Autodesk Inventor part; units mm, degrees
ref_plane "YZ Plane" through (0, 0, 0) normal (1, 0, 0) x (0, 1, 0)
ref_plane "XZ Plane" through (0, 0, 0) normal (0, 1, 0) x (-1, 0, 0)
sketch "Sketch1" plane through (0, 0, 0) normal (0, 0, 1) x (1, 0, 0)
  line L0 (0, 0) -> (98, 0)
  line L1 (98, 0) -> (98, 11.5)
  line L2 (98, 11.5) -> (0, 11.5)
  line L3 (0, 11.5) -> (0, 0)
  circle A0 centre (8, 5.75) radius 4
  arc A1 (7, 4.632) -> (7, 6.868) centre (8, 5.75) ccw
  line L4 (7, 6.868) -> (7, 4.632)
  circle A2 centre (28, 5.75) radius 4
  arc A3 (27, 4.632) -> (27, 6.868) centre (28, 5.75) ccw
  line L5 (27, 6.868) -> (27, 4.632)
  circle A4 centre (48, 5.75) radius 4
  arc A5 (47, 4.632) -> (47, 6.868) centre (48, 5.75) ccw
  line L6 (47, 6.868) -> (47, 4.632)
  circle A6 centre (68, 5.75) radius 4
  arc A7 (67, 4.632) -> (67, 6.868) centre (68, 5.75) ccw
  line L7 (67, 6.868) -> (67, 4.632)
  circle A8 centre (88, 5.75) radius 4
  arc A9 (87, 4.632) -> (87, 6.868) centre (88, 5.75) ccw
  line L8 (87, 6.868) -> (87, 4.632)
  point P0 (0, 5.75)
  dimension "d0" = 11.5
  dimension "d1" = 8
  dimension "d2" = 8
  dimension "d3" = 1.5
  dimension "d4" = 1
  dimension "d7" = 20
  dimension "d12" = 98
extrude "Extrusion1" add sketch "Sketch1" along normal blind 3 contours L3 L2 L1 L0 | A0 | L4 A1 | A2 | L5 A3 | A4 | L6 A5 | A6 | L7 A7 | A8 | L8 A9
sketch "Sketch2" plane through (0, 0, 3) normal (0, 0, 1) x (1, 0, 0)
  circle A0 centre (8, 5.75) radius 4
  arc A1 (7, 4.632) -> (7, 6.868) centre (8, 5.75) ccw
  line L0 (7, 6.868) -> (7, 4.632)
  circle A2 centre (28, 5.75) radius 4 construction
  arc A3 (27, 4.632) -> (27, 6.868) centre (28, 5.75) ccw construction
  line L1 (27, 6.868) -> (27, 4.632) construction
  line L2 (47, 6.868) -> (47, 4.632) construction
  arc A4 (47, 4.632) -> (47, 6.868) centre (48, 5.75) ccw construction
  circle A5 centre (48, 5.75) radius 4 construction
  circle A6 centre (68, 5.75) radius 4 construction
  arc A7 (67, 4.632) -> (67, 6.868) centre (68, 5.75) ccw construction
  line L3 (67, 6.868) -> (67, 4.632) construction
  line L4 (87, 6.868) -> (87, 4.632) construction
  arc A8 (87, 4.632) -> (87, 6.868) centre (88, 5.75) ccw construction
  circle A9 centre (88, 5.75) radius 4 construction
  circle A10 centre (28, 5.75) radius 4.05
  arc A11 (26.95, 4.6098) -> (26.95, 6.8902) centre (28, 5.75) ccw
  line L5 (26.95, 4.6098) -> (26.95, 6.8902)
  circle A12 centre (48, 5.75) radius 4.1
  line L6 (46.9, 4.5881) -> (46.9, 6.9119)
  arc A13 (46.9, 4.5881) -> (46.9, 6.9119) centre (48, 5.75) ccw
  circle A14 centre (68, 5.75) radius 4.15
  arc A15 (66.85, 4.5668) -> (66.85, 6.9332) centre (68, 5.75) ccw
  line L7 (66.85, 4.5668) -> (66.85, 6.9332)
  line L8 (86.8, 4.5458) -> (86.8, 6.9542)
  arc A16 (86.8, 4.5458) -> (86.8, 6.9542) centre (88, 5.75) ccw
  circle A17 centre (88, 5.75) radius 4.2
  point P0 (0, 0)
  dimension "d15" = 0.05
  dimension "d17" = 0.05
  dimension "d18" = 0.1
  dimension "d19" = 0.1
  dimension "d20" = 0.15
  dimension "d21" = 0.15
  dimension "d22" = 0.2
  dimension "d23" = 0.2
extrude "Extrusion2" add sketch "Sketch2" along normal blind 8
sketch "Sketch3" plane through (0, 0, 3) normal (0, 0, 1) x (1, 0, 0)
  circle A0 centre (8, 5.75) radius 4
  circle A1 centre (8, 5.75) radius 5
  line L0 (0, 0) -> (98, 0)
  circle A2 centre (28, 5.75) radius 5
  circle A3 centre (48, 5.75) radius 5
  circle A4 centre (68, 5.75) radius 5
  circle A5 centre (88, 5.75) radius 5
  dimension "d26" = 1
  dimension "d29" = 20
extrude "Extrusion3" add sketch "Sketch3" along normal blind 0.5 contours A0 | A1 | A2 | A3 | A4 | A5
chamfer "Chamfer1" distance 0.1 angle 45 15 edges at (4, 5.75, 11) (9.5, 5.75, 11) (7, 5.75, 11) (23.95, 5.75, 11) (29.55, 5.75, 11) (26.95, 5.75, 11) (43.9, 5.75, 11) (49.6, 5.75, 11) (46.9, 5.75, 11) (69.65, 5.75, 11) (66.85, 5.75, 11) (63.85, 5.75, 11) (83.8, 5.75, 11) (89.7, 5.75, 11) (86.8, 5.75, 11)
sketch "Sketch4" plane through (0, 0, 3) normal (0, 0, 1) x (1, 0, 0)
  line L0 (15, 8.25) -> (15, 3.25)
  line L1 (15, 3.25) -> (20, 5.75)
  line L2 (20, 5.75) -> (15, 8.25)
  line L3 (0, 11.5) -> (0, 0)
  line L4 (0, 5.75) -> (37.8806, 5.75)
  dimension "d39" = 15
  dimension "d40" = 5
  dimension "d41" = 5
extrude "Extrusion4" cut sketch "Sketch4" against normal blind 0.5
properties part number "insert_testing_3Dprint"
Work out the finished part from the listing and answer in its coordinate system (mm). A direction names the side the tool comes from. Round coordinates to 2 decimals unless told otherwise and drop trailing zeros. Write each loop counter-clockwise with the first axis right and the second up, starting at its lowest first coordinate (ties: lowest second). Pieces come first, ordered by that corner, then holes.
1) A cutting plane is placed at A-A (z = 7.75). Give the number of separate pieces and of enclosed holes in the cut face, plus the area to 3 significant figures.
2) Straight lines are drawn through the part: line 1 (Y direction, x = 88, z = 7.5); line 2 (Y direction, x = 48, z = 8.25); line 3 (Z direction, x = 13, y = 8.25). For each, find the intervals that lie inside material, in ascending order.
3) Given pin 1 Ø1.9 at (x, y) = (28, 5.75) entering from +Z; pin 2 Ø1.9 at (y, z) = (6, 6) entering from +X; pin 3 Ø5.5 at (x, y) = (18, 6.5) entering from +Z, each flat-ended and moving along its own axis, determine where each tip first touches the part or whether it passes through.
4) A cutting plane is placed at B-B (x = 48). Give the vertices of the cut face in (y, z), plus the area to 3 significant figures.
5) The mould has two halves that part along X. Classify faces 3 (the flat face through (0, 6, 1)), 4 (the cylindrical face through (9.5, 5.8, 7.1)), 5 (the flat face through (48, 0, 1)): pulls with the +X half, pulls with the -X half, needs draft (parallel to the pull), parting line crosses it, or undercut.
6) A tool of negligible diameter and unlimited length cuts with its end or side. For faces 1 (the flat face through (48, 6, 0)), 2 (the flat face through (4, 4, 3.5)), from which of +Z, -Z, +X, -X, +Y, -Y can it reach the whole face along a straight path? Write none if from no direction.
Completed:
1. separate pieces: 5
1. enclosed holes: 5
1. area: 228 mm2
2. line 1: y = 1.55 to 4.05, 7.45 to 9.95
2. line 2: y = 1.65 to 4.15, 7.35 to 9.85
2. line 3: z = 0 to 3
3. pin 1: stops at z = 3.5
3. pin 2: stops at x = 92.2
3. pin 3: stops at z = 3
4. outline: (0, 0) - (11.5, 0) - (11.5, 3) - (10.75, 3) - (10.75, 3.5) - (9.85, 3.5) - (9.85, 10.9) - (9.75, 11) - (7.45, 11) - (7.35, 10.9) - (7.35, 3.5) - (4.15, 3.5) - (4.15, 10.9) - (4.05, 11) - (1.75, 11) - (1.65, 10.9) - (1.65, 3.5) - (0.75, 3.5) - (0.75, 3) - (0, 3) - close
4. area: 77.0 mm2
5. face 3: pulls with the -X half
5. face 4: undercut
5. face 5: needs draft
6. face 1: -Z, +X, -X, +Y, -Y
6. face 2: +Z
